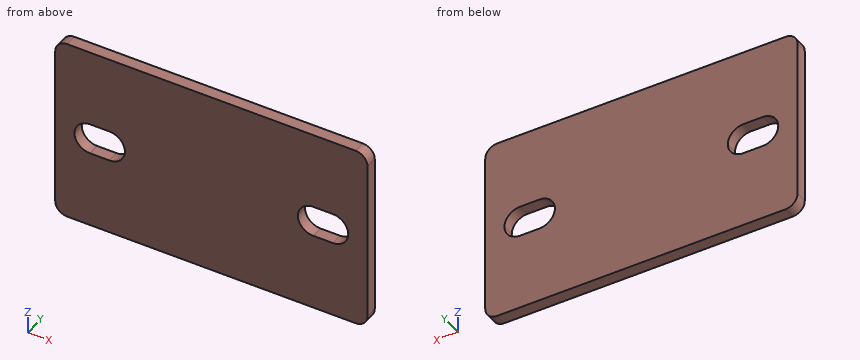
```python
from build123d import *

# Parameters (mm, degrees)
F0_W     = 130
F0_H     = 77.4
F1_DEPTH = 5
F2_R     = 5


with BuildPart() as f1:
    # F0 (on Front) → F1 (new body)
    with BuildSketch(Plane.XZ):
        Rectangle(F0_W, F0_H)
        with BuildLine():
            ThreePointArc((-36, 0), (-37.903806, -4.596194), (-42.5, -6.5))
            Line((-42.5, -6.5), (-50.5, -6.5))
            ThreePointArc((-50.5, -6.5), (-55.096194, -4.596194), (-57, 0))
            ThreePointArc((-57, 0), (-55.096194, 4.596194), (-50.5, 6.5))
            Line((-50.5, 6.5), (-42.5, 6.5))
            ThreePointArc((-42.5, 6.5), (-37.903806, 4.596194), (-36, 0))
        make_face(mode=Mode.SUBTRACT)
        with BuildLine():
            ThreePointArc((50.5, 6.5), (55.096194, 4.596194), (57, 0))
            ThreePointArc((57, 0), (55.096194, -4.596194), (50.5, -6.5))
            Line((50.5, -6.5), (42.5, -6.5))
            ThreePointArc((42.5, -6.5), (37.903806, -4.596194), (36, 0))
            ThreePointArc((36, 0), (37.903806, 4.596194), (42.5, 6.5))
            Line((42.5, 6.5), (50.5, 6.5))
        make_face(mode=Mode.SUBTRACT)
    extrude(amount=F1_DEPTH)

    # F2
    f2_edges = [f1.edges().sort_by_distance(p)[0] for p in [
        (65, -2.5, 38.7),
        (65, -2.5, -38.7),
        (-65, -2.5, -38.7),
        (-65, -2.5, 38.7),
    ]]
    fillet(f2_edges, radius=F2_R)


solid = f1.part
```
Could you check a few things on this model? Use its own coordinates, in mm. Round coordinates to 2 decimals unless told otherwise and drop trailing zeros. Write each loop counter-clockwise with the first axis right and the second up, starting at its lowest first coordinate (ties: lowest second). Pieces come first, ordered by that corner, then holes.
(1) Suppose I cut it at A-A on x = 39. Write out the boundary of the cut face in (y, z).
Findings below:
outline: (-5, -38.7) - (0, -38.7) - (0, -5.48) - (-5, -5.48) - close; (-5, 5.48) - (0, 5.48) - (0, 38.7) - (-5, 38.7) - close
(2) Suppose I cut it at C-C on z = 3.5. Write out the boundary of the cut face in (x, y).
Findings below:
outline: (-65, -5) - (-55.98, -5) - (-55.98, 0) - (-65, 0) - close; (-37.02, -5) - (37.02, -5) - (37.02, 0) - (-37.02, 0) - close; (55.98, -5) - (65, -5) - (65, 0) - (55.98, 0) - close
(3) Suppose I cut it at B-B on y = -1.7. Write out the boundary of the cut face in (x, z).
Findings below:
outline: (-65, -33.7) arc R5 ccw to (-60, -38.7) - (60, -38.7) arc R5 ccw to (65, -33.7) - (65, 33.7) arc R5 ccw to (60, 38.7) - (-60, 38.7) arc R5 ccw to (-65, 33.7) - close; hole (-50.5, -6.5) - (-42.5, -6.5) arc R6.5 ccw to (-42.5, 6.5) - (-50.5, 6.5) arc R6.5 ccw to start; hole (42.5, -6.5) - (50.5, -6.5) arc R6.5 ccw to (50.5, 6.5) - (42.5, 6.5) arc R6.5 ccw to start
(4) If I drill on probe 1 along X at (y, z) = (-2.8, 6); probe 2 along X at (y, z) = (-1.05, 4); probe 3 along Z at (x, y) = (38, -2.65), over which ranges is the centre line in solid material (lowest first)?
Findings below:
probe 1: x = -65 to -53, -40 to 40, 53 to 65
probe 2: x = -65 to -55.62, -37.38 to 37.38, 55.62 to 65
probe 3: z = -38.7 to -4.69, 4.69 to 38.7
